from build123d import *

# Parameters (mm, degrees)
BOSS_EXTRUDE1_DEPTH      = 6.5
M7_CLEARANCE_HOLE1_D     = 8
M7_CLEARANCE_HOLE1_DEPTH = 14
M7_CLEARANCE_HOLE1_TIP   = 2.403442476
FILLET1_R                = 0.5


with BuildPart() as part:
    # Sketch1 → Boss-Extrude1 (new body)
    with BuildSketch(Plane.XY):
        Polygon((-7.505553499, 0), (-3.75277675, -6.5), (3.75277675, -6.5), (7.505553499, 0), (3.75277675, 6.5), (-3.75277675, 6.5), align=None)
    extrude(amount=BOSS_EXTRUDE1_DEPTH)

    # M7 Clearance Hole1
    with Locations(Plane.XY.offset(6.5)):
        with Locations((0, 0)):
            Hole(M7_CLEARANCE_HOLE1_D / 2, depth=M7_CLEARANCE_HOLE1_DEPTH)
            with Locations((0, 0, -(M7_CLEARANCE_HOLE1_DEPTH + M7_CLEARANCE_HOLE1_TIP / 2))):  # 118° drill point
                Cone(0, M7_CLEARANCE_HOLE1_D / 2, M7_CLEARANCE_HOLE1_TIP, mode=Mode.SUBTRACT)

    # Fillet1
    fillet1_edges = [part.edges().sort_by_distance(p)[0] for p in [
        (0, -6.5, 6.5),
        (-3.75277675, 6.5, 3.25),
        (3.75277675, 6.5, 3.25),
        (7.505553499, 0, 3.25),
        (3.75277675, -6.5, 3.25),
        (-3.75277675, -6.5, 3.25),
        (-7.505553499, 0, 3.25),
        (5.629165125, -3.25, 6.5),
        (5.629165125, 3.25, 6.5),
        (0, 6.5, 6.5),
        (4, 0, 0),
        (4, 0, 6.5),
        (-5.629165125, 3.25, 6.5),
        (0, 6.5, 0),
        (5.629165125, 3.25, 0),
        (5.629165125, -3.25, 0),
        (-5.629165125, -3.25, 6.5),
        (0, -6.5, 0),
        (-5.629165125, -3.25, 0),
        (-5.629165125, 3.25, 0),
    ]]
    fillet(fillet1_edges, radius=FILLET1_R)


solid = part.part
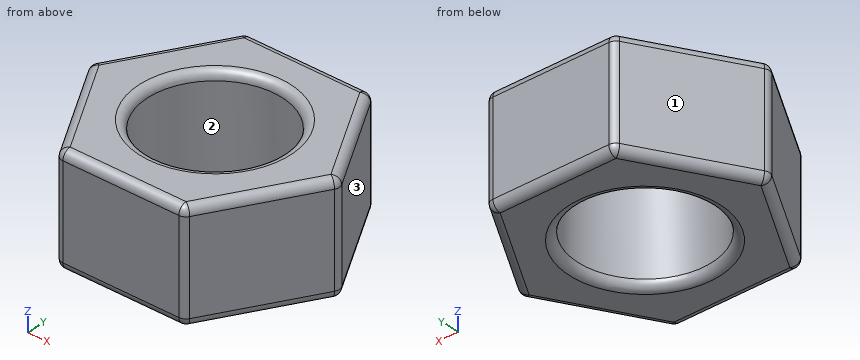
The model under review builds one solid part; all positions refer to its coordinate system, in mm. Face numbers are marked on the shaded views. Round coordinates to 2 decimals unless told otherwise and drop trailing zeros. Order: outer loops, then holes, each group sorted by start corner. A loop starts at its lowest first (then second) coordinate and runs counter-clockwise, first axis right, second up. Notation, with made-up numbers: (-35.5, 5) -> (5.5, 5) arc R9 cw to (5.5, 20) -> close; hole circle Ø1 at (71.5, 55.25). An arc over 180 degrees is marked (long way). Write item = value, one per line. Start each with the question number.
Item 1: Consider section B-B on z = 2.75. Write out the cut boundary in (x, y), plus the area to 3 significant figures.
Item 2: For line 1 along Y through (x, z) = (0, 2.05); line 2 along Y through (x, z) = (-3.5, 0.5); line 3 along X through (y, z) = (2, 3.5), list the stretches that pass through material, from the lowest coordinate up.
Item 3: Mouldability with a two-part tool opening along X and no side actions: class the marked faces 1, 2 and 3 as released by +X, released by -X, zero draft, split by the parting line, or undercut.
Item 4: Consider section A-A on x = 0. Write out the cut boundary in (y, z), plus the area to 3 significant figures.
Item 5: Clearance check with flat-ended pins moving along their axes: pin 1 Ø1 at (y, z) = (4.5, 4.5) entering from -X; pin 2 Ø2 at (x, z) = (-5, 2) entering from -Y; pin 3 Ø3 at (y, z) = (-2.5, 4.5) entering from -X. State where each tip first meets the part, or that it passes through.
Conclusion:
q1.outline = (-7.36, -0.25) -> (-3.9, -6.25) arc R0.5 ccw to (-3.46, -6.5) -> (3.46, -6.5) arc R0.5 ccw to (3.9, -6.25) -> (7.36, -0.25) arc R0.5 ccw to (7.36, 0.25) -> (3.9, 6.25) arc R0.5 ccw to (3.46, 6.5) -> (-3.46, 6.5) arc R0.5 ccw to (-3.9, 6.25) -> (-7.36, 0.25) arc R0.5 ccw to start; hole circle Ø8 at (0, 0)
q1.area = 96.0 mm2
q2.line_1 = -6.5 to -4, 4 to 6.5
q2.line_2 = -6.5 to -1.94, 1.94 to 6.5
q2.line_3 = -6.35 to -3.46, 3.46 to 6.35
q3.face_1 = released by -X
q3.face_2 = undercut
q3.face_3 = released by +X
q4.outline = (-6.5, 0.5) arc R0.5 ccw to (-6, 0) -> (-4.5, 0) arc R0.5 ccw to (-4, 0.5) -> (-4, 6) arc R0.5 ccw to (-4.5, 6.5) -> (-6, 6.5) arc R0.5 ccw to (-6.5, 6) -> close; (4, 0.5) arc R0.5 ccw to (4.5, 0) -> (6, 0) arc R0.5 ccw to (6.5, 0.5) -> (6.5, 6) arc R0.5 ccw to (6, 6.5) -> (4.5, 6.5) arc R0.5 ccw to (4, 6) -> close
q4.area = 32.1 mm2
q5.pin_1 = -5.2
q5.pin_2 = -6.07
q5.pin_3 = -6.93
